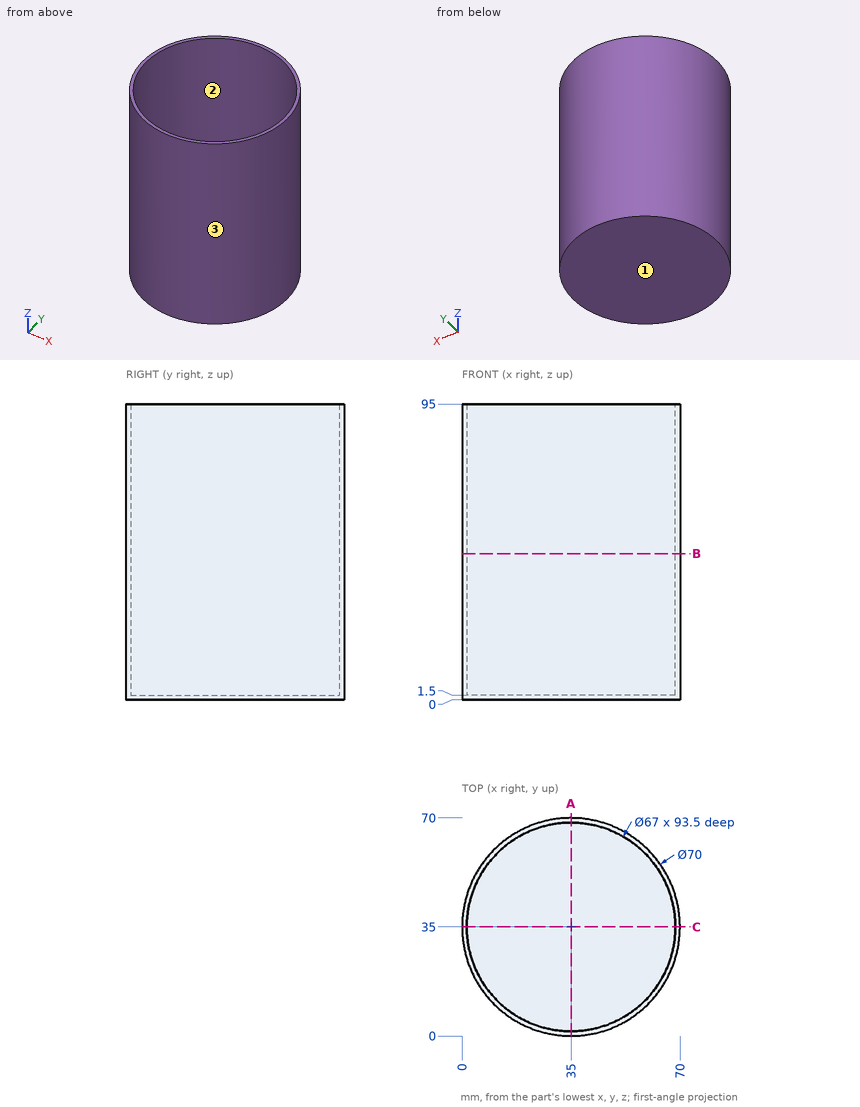
Verification items for this drawing (mm, ordinates from the low corner). Give positions to 0.01 mm unless a question says otherwise; leave off trailing zeros. Loops run counter-clockwise (first coordinate to the right, second up) from the corner with the lowest first, then second, coordinate; pieces in that order, holes last. Notation, with made-up numbers: M 21.5,32 L 68.5,32 A23 ccw 68.5,50 Z; hole C -25.75,35.25 d5. An arc over 180 degrees is marked long. Return JSON: item names as keys, results as strings. Group by question number.
1. Cross-section at A-A on x = 35. Record the boundary of the cut face in (y, z).
2. Thickness scan on L1, parallel to X at y = 35.5, z = 61.5; L2, parallel to Z at x = 33, y = 3. Record the ranges inside material, lowest first.
3. Cross-section at B-B on z = 47. Record the boundary of the cut face in (x, y).
4. Mould release check, pull along Y, two halves, no side actions. Record for the marked faces 1, 2 and 3: released by +Y, released by -Y, zero draft, split by the parting line, or undercut.
5. Go/stop test with flat-tipped pins: pin 1 (10 mm diameter, centred on y = 25.5, z = 61, fed in from +X); pin 2 (1.5 mm diameter, centred on x = 50, z = 13, fed in from -Y); pin 3 (12 mm diameter, centred on y = 13, z = 63, fed in from +X). Record where each tip stops, or that it passes through.
Return value:
{
 "1": {"outline": "M 0,0 L 70,0 L 70,95 L 68.5,95 L 68.5,1.5 L 1.5,1.5 L 1.5,95 L 0,95 Z"},
 "2": {"L1": "0 to 1.5, 68.5 to 70", "L2": "0 to 1.5"},
 "3": {"outline": "C 35,35 d70; hole C 35,35 d67"},
 "4": {"face 1": "zero draft", "face 2": "undercut", "face 3": "split by the parting line"},
 "5": {"pin 1": "x = 69.71", "pin 2": "y = 3.03", "pin 3": "x = 66.13"}
}
